```python
from build123d import *

# Parameters (mm, degrees)
F1_DEPTH = 50
F2_SIZE  = 5


with BuildPart() as f1:
    # F0 (on Front) → F1 (new body, symmetric)
    with BuildSketch(Plane.XZ):
        Polygon((26.245609, 13.570482), (0, 0), (43.497787, -25.113462), align=None)
        Polygon((43.497787, -25.113462), (0, 0), (-1.370423, -29.514605), align=None)
        Polygon((0, 50.226919), (0, 0), (26.245609, 13.570482), align=None)
        Polygon((-24.875186, 15.944123), (0, 0), (0, 50.226919), align=None)
        Polygon((-43.497791, -25.113455), (0, 0), (-24.875186, 15.944123), align=None)
        Polygon((-1.370423, -29.514605), (0, 0), (-43.497791, -25.113455), align=None)
    extrude(amount=F1_DEPTH, both=True)

    # F2
    f2_edges = [f1.edges().sort_by_distance(p)[0] for p in [
        (-43.497791, 0, -25.113455),
        (43.497787, 0, -25.113462),
        (0, 0, 50.226919),
    ]]
    chamfer(f2_edges, length=F2_SIZE)


solid = f1.part
```
Design review of the part built by this model. Coordinates are the model's own, in mm. Coordinates: 2 decimals unless noted, no trailing zeros. Loops run counter-clockwise (first coordinate to the right, second up) from the corner with the lowest first, then second, coordinate; pieces in that order, holes last. Notation, with made-up numbers: M 55.5,-24 L 100.5,-24 A28 ccw 100.5,4 Z; hole C 64.25,32.5 d10. An arc over 180 degrees is marked long. One line per question, with ' | ' between items.
(1) We need section A-A (y = -11). Give the boundary of the cut face in (x, z), and give its area (3 significant figures).
Filled in:
outline: M -41.43,-20.56 L -38.52,-25.63 L -1.37,-29.51 L 38.52,-25.6 L 41.46,-20.55 L 26.25,13.57 L 2.91,46.16 L -2.94,46.18 L -24.88,15.94 Z | area: 3,820 mm^2
(2) We need section C-C (x = -18). Give the boundary of the cut face in (y, z), and give its area (3 significant figures).
Filled in:
outline: M -50,-27.78 L 50,-27.78 L 50,25.42 L -50,25.42 Z | area: 5,320 mm^2
(3) We need section B-B (z = 26). Give the boundary of the cut face in (x, y), and give its area (3 significant figures).
Filled in:
outline: M -17.58,-50 L 17.35,-50 L 17.35,50 L -17.58,50 Z | area: 3,490 mm^2
(4) For pin 1 Ø1 at (y, z) = (-10, -1) entering from +X; pin 2 Ø2 at (x, y) = (-14, -26) entering from -Z; pin 3 Ø10 at (x, y) = (-14, 15) entering from +Z, all flat-tipped, find the tip position at first contact; note any pin that passes through.
Filled in:
pin 1: stops at x = 32.97 | pin 2: stops at z = -28.3 | pin 3: stops at z = 37.82
(5) Wall thickness on probe 1 along Z at (x, y) = (9, 34.5); probe 2 along X at (y, z) = (27, -3); probe 3 along X at (y, z) = (14, -3.5): over which ranges is each line inside the solid? List them lowest first.
Filled in:
probe 1: z = -28.5 to 37.66 | probe 2: x = -33.47 to 33.64 | probe 3: x = -33.69 to 33.86
